Source: CAD feature listing. Evaluate the final solid. Frame: model axes, mm. Give positions to 0.01 mm unless a question says otherwise; leave off trailing zeros. Order: outer loops, then holes, each group sorted by start corner. A loop starts at its lowest first (then second) coordinate and runs counter-clockwise, first axis right, second up. Notation, with made-up numbers: M -39,52.5 L 9,52.5 A25 cw 9,89.5 Z; hole C -5.75,55 d9. An arc over 180 degrees is marked long. Answer in a Markdown table with one row per item. Add a question column.
(1) Material intervals for line 1 along Y through (x, z) = (-22.5, 0.75); line 2 along X through (y, z) = (50, 0.75); line 3 along Y through (x, z) = (-29, 0.7), sorted ascending.
(2) Section query C-C, the plane x = -43. Return loops of the section in (y, z).
(3) Pin query (flat end, axial travel): P1, Ø0.5, axis at y = -23.5, z = 0.5, coming from the -X side; P2, Ø0.5, axis at y = 60.5, z = 0.5, coming from the +X side; P3, Ø0.5, axis at y = 51.5, z = 0.5, coming from the +X side. Return the tip coordinate at first contact, or that it passes through.
(4) Section query A-A, the plane z = 0.2. Count the separate pieces of the cut face and the enclosed holes in it, plus the area to 3 significant figures.
(5) Section query B-B, the plane x = -10. Return loops of the section in (y, z), plus the area to 3 significant figures.
from build123d import *

# Parameters (mm, degrees)
F1_DEPTH = 1


with BuildPart() as f1:
    # F0 (on Top) → F1 (new body)
    with BuildSketch(Plane.XY):
        with BuildLine():
            Line((-6.292982, -85.910741), (-6.292982, 54.089259))
            ThreePointArc((-6.292982, 54.089259), (-26.288129, 74.529796), (-46.283277, 54.089259))
            Line((-46.283277, 54.089259), (-46.283277, -85.910741))
            Line((-46.283277, -85.910741), (-6.292982, -85.910741))
        make_face()
        Polygon((-39.135793, 58.156283), (-37.816775, 57.748809), (-36.096451, 54.285815), (-31.550451, 52.930429), (-34.276498, 48.838314), (-33.578717, 45.068727), (-34.385781, 43.934663), (-35.333624, 49.055149), (-33.132877, 52.358728), (-36.79867, 53.451681), align=None, mode=Mode.SUBTRACT)
        Polygon((-33.571035, 43.354844), (-32.763971, 44.488907), (-29.039516, 45.054648), (-26.94571, 47.962227), (-26.847435, 46.38745), (-28.473701, 44.129124), align=None, mode=Mode.SUBTRACT)
        Polygon((-29.588758, 64.103655), (-29.478391, 59.056225), (-34.174348, 60.578728), (-37.521616, 58.704257), (-38.840633, 59.111731), (-34.281651, 61.664762), (-30.508922, 60.441584), (-30.598373, 64.532466), (-26.796919, 68.043156), (-26.805587, 66.673948), align=None, mode=Mode.SUBTRACT)
        with BuildLine():
            Line((-30.048708, 54.077201), (-27.361293, 54.621597))
            Line((-27.361293, 54.621597), (-27.047152, 49.587743))
            ThreePointArc((-27.047152, 49.587743), (-31.287939, 54.486218), (-27.133178, 59.457868))
            Line((-27.133178, 59.457868), (-27.056337, 56.245149))
            Line((-27.056337, 56.245149), (-30.742993, 55.498334))
            Line((-30.742993, 55.498334), (-30.048708, 54.077201))
        make_face(mode=Mode.SUBTRACT)
        Polygon((-25.498227, 46.435824), (-25.498227, 48.115821), (-23.230623, 45.054648), (-19.486444, 44.488301), (-18.682042, 43.355251), (-23.788412, 44.127645), align=None, mode=Mode.SUBTRACT)
        with BuildLine():
            Line((-25.498227, 49.592584), (-25.498227, 55.169558))
            Line((-25.498227, 55.169558), (-21.502735, 55.978935))
            ThreePointArc((-21.502735, 55.978935), (-22.049338, 51.877881), (-25.498227, 49.592584))
        make_face(mode=Mode.SUBTRACT)
        Polygon((-17.866638, 43.934143), (-18.67104, 45.067193), (-17.961659, 48.838314), (-21.025808, 52.930429), (-16.2674, 54.475481), (-14.564381, 57.960362), (-13.23457, 58.40398), (-15.555168, 53.655348), (-19.387565, 52.410971), (-16.897593, 49.085659), align=None, mode=Mode.SUBTRACT)
        with BuildLine():
            Line((-22.088989, 57.244058), (-25.388635, 56.97))
            Line((-25.388635, 56.97), (-25.597259, 59.481836))
            ThreePointArc((-25.597259, 59.481836), (-23.599271, 58.745248), (-22.088989, 57.244058))
        make_face(mode=Mode.SUBTRACT)
        Polygon((-13.55102, 59.352589), (-14.880832, 58.908971), (-18.361953, 60.687206), (-23.098863, 59.010709), (-23.098863, 64.103655), (-25.805607, 66.667618), (-25.796939, 68.036826), (-22.098863, 64.533824), (-22.098863, 60.425414), (-18.290102, 61.773419), align=None, mode=Mode.SUBTRACT)
    extrude(amount=F1_DEPTH)


solid = f1.part
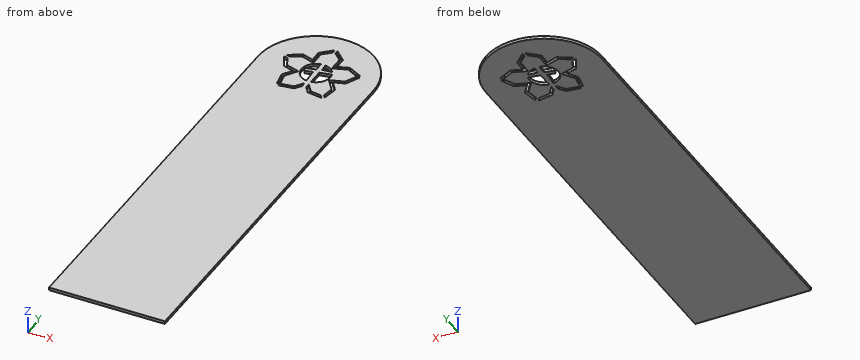
Values follow:
| question | item | result |
|---|---|---|
| 1 | line 1 | y = -85.91 to 43.93, 44.94 to 51.27, 55.78 to 57.21, 57.79 to 59.22, 64.91 to 74.17 |
| 1 | line 2 | x = -46.28 to -34.7, -33.5 to -28.4, -27.07 to -25.5, -24.17 to -18.83, -17.58 to -6.29 |
| 1 | line 3 | y = -85.91 to 44.05, 45.11 to 50.33, 54.29 to 55.85, 58.73 to 64.65, 66.01 to 74.35 |
| 2 | outline | M -85.91,0 L 65.52,0 L 65.52,1 L -85.91,1 Z |
| 3 | P1 | stops at x = -46.28 |
| 3 | P2 | stops at x = -7.12 |
| 3 | P3 | stops at x = -6.29 |
| 4 | separate pieces | 1 |
| 4 | enclosed holes | 9 |
| 4 | area | 6,110 mm² |
| 5 | outline | M -85.91,0 L 66.14,0 L 66.14,1 L -85.91,1 Z |
| 5 | area | 152 mm² |
